from build123d import *

# Parameters (mm, degrees)
SKETCH1_W           = 83.18
SKETCH1_H           = 94.48
SKETCH1_R           = 1.25
SKETCH1_R_2         = 3.5
BOSS_EXTRUDE1_DEPTH = 0.35


with BuildPart() as part:
    # Sketch1 → Boss-Extrude1 (new body)
    with BuildSketch(Plane(origin=(0, 0, 0), x_dir=(1, 0, 0), z_dir=(0, 1, 0))):
        with Locations((38.67, 44.32)):
            Rectangle(SKETCH1_W, SKETCH1_H)
        with Locations(Location((0, 88.64, 0), (0, 0, 270))):
            Circle(SKETCH1_R, mode=Mode.SUBTRACT)
        with Locations(Location((77.34, 88.64, 0), (0, 0, 270))):
            Circle(SKETCH1_R, mode=Mode.SUBTRACT)
        with Locations(Location((77.34, 0, 0), (0, 0, 270))):
            Circle(SKETCH1_R, mode=Mode.SUBTRACT)
        with Locations(Location((0, 0, 0), (0, 0, 270))):
            Circle(SKETCH1_R, mode=Mode.SUBTRACT)
        with Locations(Location((11.302, 14.24, 0), (0, 0, 270))):
            Circle(SKETCH1_R_2, mode=Mode.SUBTRACT)
        with Locations(Location((26.095, 14.24, 0), (0, 0, 270))):
            Circle(SKETCH1_R_2, mode=Mode.SUBTRACT)
        with Locations(Location((40.888, 14.24, 0), (0, 0, 270))):
            Circle(SKETCH1_R_2, mode=Mode.SUBTRACT)
        with Locations(Location((67.047, 6.248, 0), (0, 0, 270))):
            Circle(SKETCH1_R_2, mode=Mode.SUBTRACT)
        with Locations(Location((67.047, 20.938, 0), (0, 0, 270))):
            Circle(SKETCH1_R_2, mode=Mode.SUBTRACT)
        with Locations(Location((67.047, 35.628, 0), (0, 0, 270))):
            Circle(SKETCH1_R_2, mode=Mode.SUBTRACT)
        with Locations(Location((67.047, 50.318, 0), (0, 0, 270))):
            Circle(SKETCH1_R_2, mode=Mode.SUBTRACT)
        Polygon((2.08, 86.56), (60.08, 86.56), (76.192857175, 86.56), (76.192857175, 55.768), (60.08, 55.768), (60.08, 21.56), (2.08, 21.56), align=None, mode=Mode.SUBTRACT)
    extrude(amount=BOSS_EXTRUDE1_DEPTH)


solid = part.part
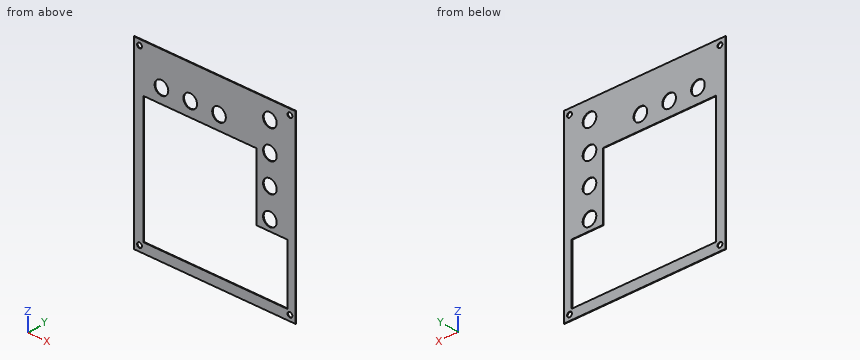
Model file for the job. Use its own axes, mm. Give positions to 0.01 mm unless a question says otherwise; leave off trailing zeros. Order: outer loops, then holes, each group sorted by start corner. A loop starts at its lowest first (then second) coordinate and runs counter-clockwise, first axis right, second up. Notation, with made-up numbers: (-7, 45.5) - (9, 45.5) arc R27 cw to (9, 72.5) - close; hole circle Ø3 at (8.5, 69.25). An arc over 180 degrees is marked (long way). Write item = value, one per line. Start each with the question number.
1. Cut at B-B, the plane z = -14.24. List the corners of the cut face in (x, y) (3 decimals).
2. Cut at D-D, the plane x = 33.5. List the corners of the cut face in (y, z), and give its area (3 significant figures).
3. Cut at A-A, the plane z = -83. List the corners of the cut face in (x, y), and give its area (3 significant figures).
4. Drop a flat-ended pin along its axis: P1, Ø6.5, axis at x = 40.888, z = -14.24, coming from the -Y side. Give the stop position or say it passes through.
5. Cut at C-C, the plane x = 77.34. List the corners of the cut face in (y, z).
6. Probe line 1 along Z through (x, y) = (77.34, 0.1); line 2 along X through (y, z) = (0.3, -50); line 3 along X through (y, z) = (0.15, -88.64). List the from-to ranges inside material, lowest first.
Taken from the geometry:
q1.outline = (-2.92, 0) - (7.802, 0) - (7.802, 0.35) - (-2.92, 0.35) - close; (14.802, 0) - (22.595, 0) - (22.595, 0.35) - (14.802, 0.35) - close; (29.595, 0) - (37.388, 0) - (37.388, 0.35) - (29.595, 0.35) - close; (44.388, 0) - (80.26, 0) - (80.26, 0.35) - (44.388, 0.35) - close
q2.outline = (0, -91.56) - (0.35, -91.56) - (0.35, -86.56) - (0, -86.56) - close; (0, -21.56) - (0.35, -21.56) - (0.35, 2.92) - (0, 2.92) - close
q2.area = 10.3 mm²
q3.outline = (-2.92, 0) - (2.08, 0) - (2.08, 0.35) - (-2.92, 0.35) - close; (76.19, 0) - (80.26, 0) - (80.26, 0.35) - (76.19, 0.35) - close
q3.area = 3.17 mm²
q4.P1 = through
q5.outline = (0, -91.56) - (0.35, -91.56) - (0.35, -89.89) - (0, -89.89) - close; (0, -87.39) - (0.35, -87.39) - (0.35, -1.25) - (0, -1.25) - close; (0, 1.25) - (0.35, 1.25) - (0.35, 2.92) - (0, 2.92) - close
q6.line_1 = -91.56 to -89.89, -87.39 to -1.25, 1.25 to 2.92
q6.line_2 = -2.92 to 2.08, 60.08 to 63.56, 70.53 to 80.26
q6.line_3 = -2.92 to -1.25, 1.25 to 76.09, 78.59 to 80.26
